The model under review builds one solid part; all positions refer to its coordinate system, in mm. A direction names the side the tool comes from. Give positions to 0.01 mm unless a question says otherwise; leave off trailing zeros. Order: outer loops, then holes, each group sorted by start corner. A loop starts at its lowest first (then second) coordinate and runs counter-clockwise, first axis right, second up. Notation, with made-up numbers: (-27.5, 53) - (0.5, 53) arc R15 cw to (0.5, 70) - close; hole circle Ø3 at (-6, -30). An arc over 180 degrees is marked (long way). Use a Markdown table: item, result. Add a question column.
```python
from build123d import *

# Parameters (mm, degrees)
SKETCH1_W       = 56.9
SKETCH1_H       = 111.95
MAINBODY_DEPTH  = 31.75
SHELL1_T        = 1.5
USBCUTOUT_REACH = 106.338
SKETCH4_W       = 11
SKETCH4_H       = 8
BNCCUTOUT_REACH = 106.338


with BuildPart() as part:
    # Sketch1 → MainBody (new body)
    with BuildSketch(Plane(origin=(0, 0, 0), x_dir=(1, 0, 0), z_dir=(0, 1, 0))):
        with Locations((-1030.101436168, 22.339371288)):
            Rectangle(SKETCH1_W, SKETCH1_H)
    extrude(amount=MAINBODY_DEPTH)

    # Shell1
    shell1_openings = [part.faces().sort_by_distance(p)[0] for p in [
        (-1058.551436168, 15.875, -22.339371288),
    ]]
    offset(amount=SHELL1_T, openings=shell1_openings, kind=Kind.INTERSECTION)

    # Sketch4 → USBCutout (cut, up to next)
    with BuildSketch(Plane(origin=(-1000.151436168, 0, 0), x_dir=(0, 0, -1), z_dir=(1, 0, 0)), mode=Mode.PRIVATE) as usbcutout_sk1:
        with Locations((63.554743949, 13.594071179)):
            Rectangle(SKETCH4_W, SKETCH4_H)
    usbcutout_tool1 = extrude(usbcutout_sk1.sketch, amount=-USBCUTOUT_REACH, mode=Mode.PRIVATE) & part.part
    add(usbcutout_tool1.solids().sort_by_distance((-1000.151436, 13.594071, -63.554744))[0], mode=Mode.SUBTRACT)

    # Sketch3 → BNCCutout (cut, up to next)
    with BuildSketch(Plane(origin=(-1000.151436168, 0, 0), x_dir=(0, 0, -1), z_dir=(1, 0, 0)), mode=Mode.PRIVATE) as bnccutout_sk1:
        with BuildLine():
            Line((-15.858242347, 20.56132), (-9.313015078, 20.56132))
            ThreePointArc((-9.313015078, 20.56132), (-12.585628712, 8.66132), (-15.858242347, 20.56132))
        make_face()
    bnccutout_tool1 = extrude(bnccutout_sk1.sketch, amount=-BNCCUTOUT_REACH, mode=Mode.PRIVATE) & part.part
    # Sketch3 → BNCCutout (cut, up to next)
    with BuildSketch(Plane(origin=(-1000.151436168, 0, 0), x_dir=(0, 0, -1), z_dir=(1, 0, 0)), mode=Mode.PRIVATE) as bnccutout_sk2:
        with BuildLine():
            Line((9.541757653, 20.56132), (16.086984922, 20.56132))
            ThreePointArc((16.086984922, 20.56132), (12.814371288, 8.66132), (9.541757653, 20.56132))
        make_face()
    bnccutout_tool2 = extrude(bnccutout_sk2.sketch, amount=-BNCCUTOUT_REACH, mode=Mode.PRIVATE) & part.part
    # Sketch3 → BNCCutout (cut, up to next)
    with BuildSketch(Plane(origin=(-1000.151436168, 0, 0), x_dir=(0, 0, -1), z_dir=(1, 0, 0)), mode=Mode.PRIVATE) as bnccutout_sk3:
        with BuildLine():
            Line((34.941757653, 20.56132), (41.486984922, 20.56132))
            ThreePointArc((41.486984922, 20.56132), (38.214371288, 8.66132), (34.941757653, 20.56132))
        make_face()
    bnccutout_tool3 = extrude(bnccutout_sk3.sketch, amount=-BNCCUTOUT_REACH, mode=Mode.PRIVATE) & part.part
    add(bnccutout_tool1.solids().sort_by_distance((-1000.151436, 14.873929, 12.585629))[0], mode=Mode.SUBTRACT)
    add(bnccutout_tool2.solids().sort_by_distance((-1000.151436, 14.873929, -12.814371))[0], mode=Mode.SUBTRACT)
    add(bnccutout_tool3.solids().sort_by_distance((-1000.151436, 14.873929, -38.214371))[0], mode=Mode.SUBTRACT)


solid = part.part
```
Q1. Draft analysis for pull direction Y (two halves, no side actions). For faces 1 (the flat face through (-1030, 0, -23)), 2 (the cylindrical face through (-1000.891, 8.666, 12.352)), 3 (the flat face through (-1030, 33.25, -23)), 4 (the flat face through (-1030, 16, -79.814)), state which applies: pulls with the +Y half, pulls with the -Y half, needs draft (parallel to the pull), parting line crosses it, or undercut.
Q2. We need section C-C (y = 12). Write out the cut boundary in (x, z), plus the area to 3 significant figures.
Q3. Wall thickness on probe 1 along Z at (x, y) = (-1029.5, 16.5); probe 2 along Y at (x, z) = (-1011.5, -25); probe 3 along X at (y, z) = (29, -3): over which ranges is each line inside the solid? List them lowest first.
Q4. Clearance check with flat-ended pins moving along their axes: P1, Ø4, axis at y = 15.5, z = 21.5, coming from the -X side; P2, Ø10, axis at y = 15.06, z = -12.81, coming from the -X side. State where each tip first meets the part, or that it passes through.
Q5. We need section A-A (x = -1008). Write out the cut boundary in (y, z).
Q6. Machinability: for faces 5 (the flat face through (-1001.651, 16, -22)), 6 (the flat face through (-1058.551, 33, -22)), which of the approach directions +Z, -Z, +X, -X, +Y, -Y give a long, thin tool a straight path to every point of the face, cutting with its end or side? Answer none if there is none.
Q7. We need section B-B (z = -67). Write out the cut boundary in (x, y).
Q8. We need section D-D (y = 28). Write out the cut boundary in (x, z), plus the area to 3 significant figures.
Here are the results:
| question | item | result |
|---|---|---|
| 1 | face 1 | undercut |
| 1 | face 2 | undercut |
| 1 | face 3 | pulls with the +Y half |
| 1 | face 4 | needs draft |
| 2 | outline | (-1058.55, -79.81) - (-1000.15, -79.81) - (-1000.15, -69.05) - (-1001.65, -69.05) - (-1001.65, -78.31) - (-1058.55, -78.31) - close; (-1058.55, 33.64) - (-1001.65, 33.64) - (-1001.65, 18.21) - (-1000.15, 18.21) - (-1000.15, 35.14) - (-1058.55, 35.14) - close; (-1001.65, -58.05) - (-1000.15, -58.05) - (-1000.15, -43.83) - (-1001.65, -43.83) - close; (-1001.65, -32.59) - (-1000.15, -32.59) - (-1000.15, -18.43) - (-1001.65, -18.43) - close; (-1001.65, -7.19) - (-1000.15, -7.19) - (-1000.15, 6.97) - (-1001.65, 6.97) - close |
| 2 | area | 276 mm2 |
| 3 | probe 1 | -79.81 to -78.31, 33.64 to 35.14 |
| 3 | probe 2 | -1.5 to 0, 31.75 to 33.25 |
| 3 | probe 3 | -1001.65 to -1000.15 |
| 4 | P1 | x = -1001.65 |
| 4 | P2 | through |
| 5 | outline | (-1.5, -79.81) - (33.25, -79.81) - (33.25, 35.14) - (-1.5, 35.14) - close; hole (0, -78.31) - (31.75, -78.31) - (31.75, 33.64) - (0, 33.64) - close |
| 6 | face 5 | -X |
| 6 | face 6 | +Z, -Z, -X, +Y, -Y |
| 7 | outline | (-1058.55, -1.5) - (-1000.15, -1.5) - (-1000.15, 9.59) - (-1001.65, 9.59) - (-1001.65, 0) - (-1058.55, 0) - close; (-1058.55, 31.75) - (-1001.65, 31.75) - (-1001.65, 17.59) - (-1000.15, 17.59) - (-1000.15, 33.25) - (-1058.55, 33.25) - close |
| 8 | outline | (-1058.55, -79.81) - (-1000.15, -79.81) - (-1000.15, 35.14) - (-1058.55, 35.14) - (-1058.55, 33.64) - (-1001.65, 33.64) - (-1001.65, -78.31) - (-1058.55, -78.31) - close |
| 8 | area | 343 mm2 |
